Input: part model. Units: mm. Frame: model coordinates. A direction names the side the tool comes from. Give positions to 0.01 mm unless a question says otherwise; leave off trailing zeros. Loops run counter-clockwise (first coordinate to the right, second up) from the corner with the lowest first, then second, coordinate; pieces in that order, holes last. Notation, with made-up numbers: (89.25, -35.5) - (133.25, -35.5) arc R7 ccw to (133.25, -24.5) - close; hole circle Ø7 at (34, 9.25). An arc over 180 degrees is marked (long way). Answer as a JSON object with one key per item and string values. Group by question number.
(1) Material intervals for L1, parallel to Z at x = -14, y = 0; L2, parallel to Y at x = -45.5, z = 0; L3, parallel to Z at x = -19, y = 1.5, sorted ascending.
(2) Mould query, pull axis X, two halves, no side actions, for faces 5 (the flat face through (-17.381, 13.82, -9.22)), 6 (the cylindrical face through (-62.86, 9.98, 5.19)), 7 (the cylindrical face through (-38.507, 13.087, 7.33)). Classes: +X half, -X half, draft (parallel to the pull), parting line (faces both ways), or undercut.
(3) Pin query (flat end, axial travel): P1, Ø6.5, axis at y = 12.5, z = -8.5, coming from the +X side; P2, Ø11, axis at y = 1, z = -5.5, coming from the -X side; P3, Ø1.5, axis at x = -27, z = 8.5, coming from the -Y side; P4, Ø12, axis at x = -37, z = 9.5, coming from the +Y side. Return the tip coordinate at first contact, or that it passes through.
(4) Section query A-A (z = 0). Return loops of the section in (x, y), plus the area to 3 significant figures.
(5) Section query D-D (y = 0). Count the separate pieces of the cut face and the enclosed holes in it, plus the area to 3 significant figures.
(6) Section query C-C (x = -57.5). Return loops of the section in (y, z).
(7) Access query for faces 1 (the cylindrical face through (-14.85, -8.13, -1.07)), 2 (the conical face through (-28.8, -4.65, 14.77)), 3 (the cylindrical face through (-39, 0, -15)), 4 (the cylindrical face through (-38.51, -12.89, 7.67)). Directions: +Z, -Z, +X, -X, +Y, -Y. A direction counts if a zero-diameter tool reaches every point of the face in a straight line with its end or side. Return the directions, or none.
(8) Section query B-B (x = -41). Return loops of the section in (y, z).
```python
from build123d import *

# Parameters (mm, degrees)
F3_D           = 3.5
F3_START       = 12.3805311
F3_CBORE_D     = 8
F3_CBORE_DEPTH = 5


with BuildPart() as f1:
    # F0 (on Front) → F1 (revolve)
    with BuildSketch(Plane.XZ):
        Polygon((-12.3805310677, 8.2), (-12.3805310677, 25), (-17.3805310677, 25), (-29.3805310677, 15), (-47.3805310677, 15), (-59.3805310677, 25), (-64.3805310677, 25), (-64.3805310677, 11.25), (-61.3805310677, 11.25), (-61.3805310677, 8.2), (-31.3805310677, 8.2), (-31.3805310677, 5), (-17.3805310677, 5), (-17.3805310677, 8.2), align=None)
    revolve(axis=Axis((6.6371694137, 0, 0), (1, 0, 0)))

    # F3 (through all)
    # its depths count from where the whole tool has entered the part; down to there all is cleared
    with Locations(Plane.YZ.offset(-F3_START)):
        with Locations((0, 15), (-12.9903810568, -7.5), (12.9903810568, -7.5)):
            CounterBoreHole(F3_D / 2, F3_CBORE_D / 2, F3_CBORE_DEPTH)


solid = f1.part
```
Recorded:
{
 "1": {"L1": "z = -25 to -8.2, 8.2 to 11, 19 to 25", "L2": "y = -15 to -8.2, 8.2 to 15", "L3": "z = -23.6 to -4.77, 4.77 to 14.1, 15.9 to 23.6"},
 "2": {"face 5": "+X half", "face 6": "draft", "face 7": "undercut"},
 "3": {"P1": "stops at x = -12.38", "P2": "stops at x = -61.38", "P3": "stops at y = -15.53", "P4": "stops at y = 14.59"},
 "4": {"outline": "(-64.38, -25) - (-59.38, -25) - (-47.38, -15) - (-29.38, -15) - (-17.38, -25) - (-12.38, -25) - (-12.38, -8.2) - (-17.38, -8.2) - (-17.38, -5) - (-31.38, -5) - (-31.38, -8.2) - (-61.38, -8.2) - (-61.38, -11.25) - (-64.38, -11.25) - close; (-64.38, 11.25) - (-61.38, 11.25) - (-61.38, 8.2) - (-31.38, 8.2) - (-31.38, 5) - (-17.38, 5) - (-17.38, 8.2) - (-12.38, 8.2) - (-12.38, 25) - (-17.38, 25) - (-29.38, 15) - (-47.38, 15) - (-59.38, 25) - (-64.38, 25) - close", "area": "1,220 mm^2"},
 "5": {"separate pieces": "4", "enclosed holes": "0", "area": "1,050 mm^2"},
 "6": {"outline": "circle Ø46.87 at (0, 0); hole circle Ø3.5 at (-12.99, -7.5); hole circle Ø16.4 at (0, 0); hole circle Ø3.5 at (0, 15); hole circle Ø3.5 at (12.99, -7.5)"},
 "7": {"face 1": "+X", "face 2": "none", "face 3": "-Z", "face 4": "-Y"},
 "8": {"outline": "(-13.78, -5.94) arc R1.75 cw to (-12.03, -8.96) arc R15 ccw to (12.03, -8.96) arc R1.75 cw to (13.78, -5.94) arc R15 ccw to (1.75, 14.9) arc R1.75 cw to (-1.75, 14.9) arc R15 ccw to start; hole circle Ø16.4 at (0, 0)"}
}
